Can you work these out from the model? Positions are in its coordinate system, mm. A direction names the side the tool comes from. Round coordinates to 2 decimals unless told otherwise and drop trailing zeros. Loops run counter-clockwise (first coordinate to the right, second up) from the corner with the lowest first, then second, coordinate; pieces in that order, holes last.
from build123d import *

# Parameters (mm, degrees)
PAD004_DEPTH          = 7.5
PAD003_DEPTH          = 10
PAD002_DEPTH          = 20
CLONE_ROLL_ANGLE      = 90
CLONE_PLACEMENT_ANGLE = 180
SKETCH_R              = 14
PAD_DEPTH             = 8
FILLET_R              = 4
CHAMFER_SIZE          = 3
PAD001_DEPTH          = 5


with BuildPart() as hookpad001:
    # Sketch004 → Pad004 (new body, symmetric)
    with BuildSketch(Plane.YZ):
        with BuildLine():
            Line((-40, 0), (-40, 12))
            ThreePointArc((-39.326335, 13.626354), (-39.82492, 12.880177), (-40, 12))
            Line((-39.326335, 13.626354), (-35.759843, 17.192846))
            ThreePointArc((-35.759843, 17.192846), (-35.336431, 19.068073), (-36.847811, 20.256133))
            ThreePointArc((-36.847811, 20.256133), (-43.259533, 18.162919), (-46, 12))
            Line((-46, 0), (-46, 12))
            Line((-40, 0), (-46, 0))
        make_face()
    extrude(amount=PAD004_DEPTH, both=True)


with BuildPart() as printbolthead001:
    # Sketch003 → Pad003 (new body)
    with BuildSketch(Plane.XY):
        with BuildLine():
            ThreePointArc((-3.535526, 3.535542), (-1.8e-05, -5), (3.535551, 3.535517))
            Line((2.071068, 5), (3.535551, 3.535517))
            Line((-2.071068, 5), (2.071068, 5))
            Line((-3.535526, 3.535542), (-2.071068, 5))
        make_face()
    extrude(amount=PAD003_DEPTH)


with BuildPart() as clone_of_printboltslot:
    # Sketch002 → Pad002 (new body)
    with BuildSketch(Plane.XY):
        with BuildLine():
            ThreePointArc((-1.414208, 1.414219), (1e-06, -2), (1.414206, 1.414221))
            Line((0.828427, 2), (1.414206, 1.414221))
            Line((-0.828427, 2), (0.828427, 2))
            Line((-1.414208, 1.414219), (-0.828427, 2))
        make_face()
    extrude(amount=-PAD002_DEPTH)

    # Fusion001: union PrintBoltHead001
    add(printbolthead001.part)


with BuildPart() as clone_of_printboltslot_1:
    # Clone roll: moved
    add(clone_of_printboltslot.part.rotate(Axis((0, 0, 0), (1, 0, 0)), CLONE_ROLL_ANGLE))


with BuildPart() as clone_of_printboltslot_2:
    # Clone placement: moved
    add(clone_of_printboltslot_1.part.moved(Location((0, -15, 15))).rotate(Axis((0, -15, 15), (0, 0, 1)), CLONE_PLACEMENT_ANGLE))


with BuildPart() as mainchamfer:
    # Sketch → Pad (new body)
    with BuildSketch(Plane.XY):
        with BuildLine():
            Line((-24, -1e-06), (-24, -46))
            Line((-24, -46), (24, -46))
            Line((24, -46), (24, -1e-06))
            ThreePointArc((24, -1e-06), (0, 24), (-24, -1e-06))
        make_face()
        Circle(SKETCH_R, mode=Mode.SUBTRACT)
    extrude(amount=PAD_DEPTH)

    # Fillet
    fillet_edges = [mainchamfer.edges().sort_by_distance(p)[0] for p in [
        (24, -23, 8),
    ]]
    fillet(fillet_edges, radius=FILLET_R)

    # Chamfer
    chamfer_edges = [mainchamfer.edges().sort_by_distance(p)[0] for p in [
        (24, -23, 0),
    ]]
    chamfer(chamfer_edges, length=CHAMFER_SIZE)


with BuildPart() as hook:
    # Sketch001 → Pad001 (new body)
    with BuildSketch(Plane(origin=(0, -14, 8), x_dir=(1, 0, 0), z_dir=(0, -1, 0))):
        with BuildLine():
            ThreePointArc((19, 0), (0, 19), (-19, 0))
            Line((-19, 0), (19, 0))
        make_face()
    extrude(amount=PAD001_DEPTH)

    # Fusion: union MainChamfer
    add(mainchamfer.part)

    # Cut: cut Clone of PrintBoltSlot
    add(clone_of_printboltslot_2.part, mode=Mode.SUBTRACT)

    # Fusion002: union HookPad001
    add(hookpad001.part)


solid = hook.part
(1) If we section it at D-D, the plane z = 23.25: List the corners of the cut face in (x, y) for me, then the cut area to 3 significant figures.
Worked answers:
outline: (-11.33, -19) - (11.33, -19) - (11.33, -14) - (-11.33, -14) - close
area: 113 mm2
(2) If we mould it in two halves opening along Z, with no side actions, what happens to faces 1 (the cylindrical face through (0.11, -39.82, 12.89)), 2 (the cylindrical face through (0.165, -14.507, 10.003)), 3 (the cylindrical face through (0.105, -43.187, 18.228)), 4 (the flat face through (0, -19, 18))? For each: released by +Z, released by -Z, zero draft, split by the parting line, or undercut.
Worked answers:
face 1: undercut
face 2: undercut
face 3: released by +Z
face 4: zero draft
(3) If we section it at C-C, the plane y = -17.5: List the corners of the cut face in (x, z) for me, then the cut area to 3 significant figures.
Worked answers:
outline: (-24, 3) - (-21, 0) - (21, 0) - (24, 3) - (24, 4) arc R4 ccw to (20, 8) - (19, 8) arc R19 ccw to (-19, 8) - (-20, 8) arc R4 ccw to (-24, 4) - close; hole (-1.41, 16.41) arc R2 ccw (long way) to (1.41, 16.41) - (0.83, 17) - (-0.83, 17) - close
area: 922 mm2
(4) If I drill on line 1 (X direction, y = 0, z = 3.75); line 2 (Z direction, x = 0, y = -14.15); line 3 (Y direction, x = 0, z = 3.75), over which ranges is the centre line in solid material (lowest first)?
Worked answers:
line 1: x = -24 to -14, 14 to 24
line 2: z = 0 to 10, 20 to 27
line 3: y = -46 to -14, 14 to 24
(5) If we section it at B-B, the plane z = 15: List the corners of the cut face in (x, y) for me.
Worked answers:
outline: (-17.66, -19) - (-2, -19) - (-2, -15) - (-5, -15) - (-5, -14) - (-17.66, -14) - close; (-7.5, -45.44) - (7.5, -45.44) - (7.5, -37.95) - (-7.5, -37.95) - close; (2, -19) - (17.66, -19) - (17.66, -14) - (5, -14) - (5, -15) - (2, -15) - close
(6) Will these pins go through, and if not, where does the flat tip stop? P1, Ø3, axis at x = 17.5, y = -16, coming from the +Z side; P2, Ø6, axis at x = 9.5, y = -1.5, coming from the -Z side; P3, Ø8.5, axis at y = -43, z = 14.5, coming from the -X side; P4, Ø3, axis at x = 0, z = 15, coming from the +Y side.
Worked answers:
P1: stops at z = 18.25
P2: passes through
P3: stops at x = -7.5
P4: stops at y = -36.45
(7) If we section it at A-A, the plane y = -4: List the corners of the cut face in (x, z) for me, then the cut area to 3 significant figures.
Worked answers:
outline: (-24, 3) - (-21, 0) - (-13.42, 0) - (-13.42, 8) - (-20, 8) arc R4 ccw to (-24, 4) - close; (13.42, 0) - (21, 0) - (24, 3) - (24, 4) arc R4 ccw to (20, 8) - (13.42, 8) - close
area: 153 mm2
(8) For faces 5 (the flat face through (-23, -23, 2)), 6 (the flat face through (-2.2, -15, 15.1)), 7 (the flat face through (-4.5, -14, 17.6)), 8 (the flat face through (0, -40, 10)), which set-ups out of +Z, -Z, +X, -X, +Y, -Y let a thin tool reach every point of the face, with its end or its side?
Worked answers:
face 5: -Z, -X, +Y, -Y
face 6: +Y
face 7: +Z, +X, -X, +Y
face 8: +X, -X
